```python
from build123d import *

# Parameters (mm, degrees)
SKETCH1_R           = 45
SKETCH1_R_2         = 2
SKETCH1_W           = 20.2
SKETCH1_H           = 40.5
BOSS_EXTRUDE1_DEPTH = 5
SKETCH2_W           = 7.9
SKETCH2_H           = 15
CUT_EXTRUDE1_DEPTH  = 10
CUT_EXTRUDE2_DEPTH  = 10


with BuildPart() as part:
    # Sketch1 → Boss-Extrude1 (new body)
    with BuildSketch(Plane.XY):
        Circle(SKETCH1_R)
        with Locations((42.5, 0)):
            Circle(SKETCH1_R_2, mode=Mode.SUBTRACT)
        with Locations((0, -42.5)):
            Circle(SKETCH1_R_2, mode=Mode.SUBTRACT)
        with Locations((-42.5, 0)):
            Circle(SKETCH1_R_2, mode=Mode.SUBTRACT)
        with Locations((0, 42.5)):
            Circle(SKETCH1_R_2, mode=Mode.SUBTRACT)
        with Locations((0, 10.15)):
            Rectangle(SKETCH1_W, SKETCH1_H, mode=Mode.SUBTRACT)
    extrude(amount=BOSS_EXTRUDE1_DEPTH)

    # Sketch2 → Cut-Extrude1 (cut)
    with BuildSketch(Plane(origin=(0, 0, 0), x_dir=(-1, 0, 0), z_dir=(0, 0, -1))):
        with Locations((0, -17.6)):
            Rectangle(SKETCH2_W, SKETCH2_H)
    extrude(amount=-CUT_EXTRUDE1_DEPTH, mode=Mode.SUBTRACT)

    # Sketch3 → Cut-Extrude2 (cut)
    with BuildSketch(Plane(origin=(0, 0, 0), x_dir=(-1, 0, 0), z_dir=(0, 0, -1))):
        with BuildLine():
            Line((-19, 18), (-19, -8))
            ThreePointArc((-19, -8), (-23, -12), (-27, -8))
            Line((-27, -8), (-27, 18))
            ThreePointArc((-27, 18), (-23, 22), (-19, 18))
        make_face()
    extrude(amount=-CUT_EXTRUDE2_DEPTH, mode=Mode.SUBTRACT)


solid = part.part
```
Work out the finished part from the listing and answer in its coordinate system (mm). A direction names the side the tool comes from. Round coordinates to 2 decimals unless told otherwise and drop trailing zeros. Write each loop counter-clockwise with the first axis right and the second up, starting at its lowest first coordinate (ties: lowest second). Pieces come first, ordered by that corner, then holes.
1) Consider probe 1 along Y at (x, z) = (0, 3.25); probe 2 along X at (y, z) = (15, 1.1); probe 3 along X at (y, z) = (12, 0.9). Determine where each line is inside the solid, lowest interval first.
2) Which of the six approach directions +Z, -Z, +X, -X, +Y, -Y give full straight-line access (tool end or side, diameter ignored) to faces 1 (the face through (-10.1, 10, 2)), 2 (the face through (-11, 1, 0))?
3) Determine the mould class of faces 3 (the face through (0, 30.4, 2)), 4 (the face through (20.765, -39.923, 2.465)), 5 (the face through (-11, 1, 5)) for opening direction Y: pulls with the +Y half, pulls with the -Y half, needs draft (parallel to the pull), parting line crosses it, or undercut.
4) Flat-ended cylindrical pins translate along their axes: P1, Ø2.5, axis at x = 42.5, y = 0, coming from the +Z side; P2, Ø2.5, axis at y = 11.5, z = 3, coming from the -X side; P3, Ø1, axis at y = 4, z = 3, coming from the +X side; P4, Ø1.5, axis at x = -6.5, z = 2.5, coming from the +Y side. Find the tip coordinate at first contact, or state that the pin passes through.
5) A cutting plane is placed at C-C on x = 23. Determine the outline of the cut face in (y, z).
6) A cutting plane is placed at A-A on y = 0. Determine the outline of the cut face in (x, z).
7) A cutting plane is placed at B-B on z = 3.35. Determine the outline of the cut face in (x, y), and give its area (3 significant figures).
8) A cutting plane is placed at D-D on y = 42.5. Determine the outline of the cut face in (x, z), and give its area (3 significant figures).
Entries:
1. probe 1: y = -45 to -44.5, -40.5 to -25.1, 30.4 to 40.5, 44.5 to 45
1. probe 2: x = -42.43 to -10.1, 10.1 to 19, 27 to 42.43
1. probe 3: x = -43.37 to -10.1, 10.1 to 19, 27 to 43.37
2. face 1: +Z, -Z
2. face 2: -Z, +X, -X, +Y, -Y
3. face 3: undercut
3. face 4: parting line crosses it
3. face 5: needs draft
4. P1: passes through
4. P2: stops at x = -43.82
4. P3: stops at x = 44.86
4. P4: stops at y = 44.63
5. outline: (-38.68, 0) - (-12, 0) - (-12, 5) - (-38.68, 5) - close; (22, 0) - (38.68, 0) - (38.68, 5) - (22, 5) - close
6. outline: (-45, 0) - (-44.5, 0) - (-44.5, 5) - (-45, 5) - close; (-40.5, 0) - (-10.1, 0) - (-10.1, 5) - (-40.5, 5) - close; (10.1, 0) - (19, 0) - (19, 5) - (10.1, 5) - close; (27, 0) - (40.5, 0) - (40.5, 5) - (27, 5) - close; (44.5, 0) - (45, 0) - (45, 5) - (44.5, 5) - close
7. outline: circle Ø90 at (0, 0); hole circle Ø4 at (-42.5, 0); hole (-10.1, -10.1) - (-3.95, -10.1) - (-3.95, -25.1) - (3.95, -25.1) - (3.95, -10.1) - (10.1, -10.1) - (10.1, 30.4) - (-10.1, 30.4) - close; hole circle Ø4 at (0, -42.5); hole circle Ø4 at (0, 42.5); hole (19, -8) arc R4 ccw to (27, -8) - (27, 18) arc R4 ccw to (19, 18) - close; hole circle Ø4 at (42.5, 0)
7. area: 5,120 mm2
8. outline: (-14.79, 0) - (-2, 0) - (-2, 5) - (-14.79, 5) - close; (2, 0) - (14.79, 0) - (14.79, 5) - (2, 5) - close
8. area: 128 mm2
